Design review of the part built by this model. Coordinates are the model's own, in mm. Face numbers are marked on the shaded views. A direction names the side the tool comes from. Round coordinates to 2 decimals unless told otherwise and drop trailing zeros. Loops run counter-clockwise (first coordinate to the right, second up) from the corner with the lowest first, then second, coordinate; pieces in that order, holes last. Notation, with made-up numbers: (70.25, 63) - (126.25, 63) arc R26 cw to (126.25, 88) - close; hole circle Ø3 at (59, -31.75). An arc over 180 degrees is marked (long way). Use one line per item in the form item = value. Start each with the question number.
(1) We need section C-C, the plane z = 61. Write out the cut boundary in (x, y), then the cut area to 3 significant figures.
(2) For pin 1 (3.5 mm diameter, centred on x = 0, z = 115, fed in from -Y); pin 2 (1.8 mm diameter, centred on x = -1, y = -5, fed in from +Z); pin 3 (1.5 mm diameter, centred on y = -0.5, z = 73.5, fed in from +X); pin 4 (4 mm diameter, centred on x = -1.5, z = 5, fed in from -Y), all flat-tipped, find the tip position at first contact; note any pin that passes through.
(3) Wall thickness on probe 1 along Z at (x, y) = (-0.25, -1.25); probe 2 along Z at (x, y) = (-1.25, -0.75); probe 3 along Y at (x, z) = (1.25, 5.5): over which ranges is each line inside the solid? List them lowest first. Write a range as [from, to].
(4) Machinability: for the marked faces 1 and 2, which of the approach directions +Z, -Z, +X, -X, +Y, -Y give a long, thin tool a straight path to every point of the face, cutting with its end or side? Answer none if there is none.
(5) We need section B-B, the plane y = -1. Write out the cut boundary in (x, z).
(6) We need section A-A, the plane z = 0. Write out the cut boundary in (x, y), then the cut area to 3 significant figures.
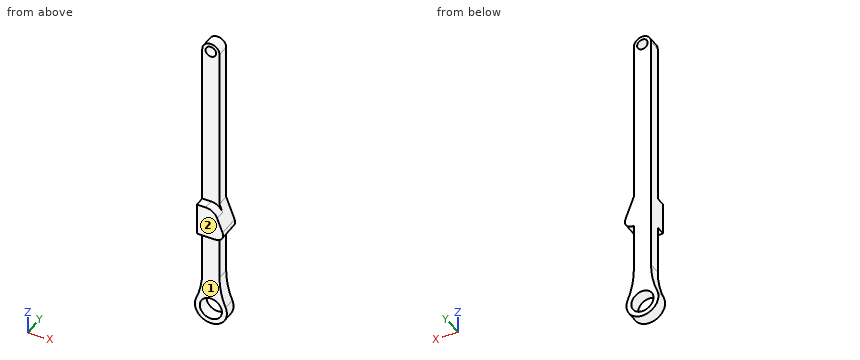
from build123d import *

# Parameters (mm, degrees)
F0_R          = 4.5
F0_R_2        = 2.15
F1_DEPTH      = 2.5
F3_DEPTH      = 4
F3_DEPTH_BACK = 5
F4_R          = 5
F5_R          = 3


with BuildPart() as f1:
    # F0 (on Front) → F1 (new body, symmetric)
    with BuildSketch(Plane.XZ):
        with BuildLine():
            ThreePointArc((-3.5, 15), (-4.13112804, 8.626225608), (-6, 2.5))
            ThreePointArc((-6, 2.5), (0, -6.5), (6, 2.5))
            ThreePointArc((6, 2.5), (4.13112804, 8.626225608), (3.5, 15))
            Line((3.5, 15), (3.5, 115))
            ThreePointArc((3.5, 115), (0, 118.5), (-3.5, 115))
            Line((-3.5, 115), (-3.5, 15))
        make_face()
        Circle(F0_R, mode=Mode.SUBTRACT)
        with Locations((0, 115)):
            Circle(F0_R_2, mode=Mode.SUBTRACT)
    extrude(amount=F1_DEPTH, both=True)

    # F2 (on face) → F3 (join, two sides)
    with BuildSketch(Plane.XZ.offset(2.5)) as f3_sk:
        Polygon((3.5, 48), (-3.5, 48), (-3.5, 35), (3.5, 35), (8.5, 35), align=None)
    extrude(amount=F3_DEPTH)
    extrude(f3_sk.sketch, amount=-F3_DEPTH_BACK)

    # F4
    f4_edges = [f1.edges().sort_by_distance(p)[0] for p in [
        (3.5, -4.5, 48),
    ]]
    fillet(f4_edges, radius=F4_R)

    # F5
    f5_edges = [f1.edges().sort_by_distance(p)[0] for p in [
        (8.5, -2, 35),
    ]]
    fillet(f5_edges, radius=F5_R)


solid = f1.part
Data:
q1.outline = (-3.5, -2.5) - (3.5, -2.5) - (3.5, 2.5) - (-3.5, 2.5) - close
q1.area = 35.0 mm^2
q2.pin_1 = through
q2.pin_2 = 48
q2.pin_3 = 3.5
q2.pin_4 = -2.5
q3.probe_1 = [-6.5, -4.49], [4.49, 112.86], [117.14, 118.49]
q3.probe_2 = [-6.38, -4.32], [4.32, 113.25], [116.75, 118.27]
q3.probe_3 = [-2.5, 2.5]
q4.face_1 = -Z, +X, -X, -Y
q4.face_2 = +Z, -Z, +X, -X, -Y
q5.outline = (-6, 2.5) arc R6.5 ccw (long way) to (6, 2.5) arc R32.5 cw to (3.5, 15) - (3.5, 35) - (4.13, 35) arc R3 ccw to (6.93, 39.08) - (3.5, 48) - (3.5, 115) arc R3.5 ccw to (-3.5, 115) - (-3.5, 15) arc R32.5 cw to start; hole circle Ø9 at (0, 0); hole circle Ø4.3 at (0, 115)
q6.outline = (-6.5, -2.5) - (-4.5, -2.5) - (-4.5, 2.5) - (-6.5, 2.5) - close; (4.5, -2.5) - (6.5, -2.5) - (6.5, 2.5) - (4.5, 2.5) - close
q6.area = 20.0 mm^2
